from build123d import *

# Parameters (mm, degrees)
SKETCH2_R           = 19.15
BOSS_EXTRUDE1_DEPTH = 25.15
SKETCH3_R           = 1.5
SKETCH3_R_2         = 3.7
CUT_EXTRUDE1_DEPTH  = 5.15
SKETCH4_R           = 7.5
BOSS_EXTRUDE2_DEPTH = 4.5
SKETCH5_R           = 4
CUT_EXTRUDE2_DEPTH  = 4.5
FILLET1_R           = 1


with BuildPart() as part:
    # Sketch2 → Boss-Extrude1 (new body)
    with BuildSketch(Plane.XY):
        with Locations(Location((0, 0, 0), (0, 0, 180))):
            Circle(SKETCH2_R)
    extrude(amount=BOSS_EXTRUDE1_DEPTH)

    # Sketch3 → Cut-Extrude1 (cut)
    with BuildSketch(Plane.XY.offset(25.15)):
        with Locations((11.66726189, 11.66726189)):
            Circle(SKETCH3_R)
        with Locations((-11.66726189, -11.66726189)):
            Circle(SKETCH3_R)
        with Locations((11.66726189, -11.66726189)):
            Circle(SKETCH3_R)
        with Locations((-11.66726189, 11.66726189)):
            Circle(SKETCH3_R)
        with Locations((0, 19.15)):
            Circle(SKETCH3_R_2)
        with Locations((0, -19.15)):
            Circle(SKETCH3_R_2)
        with Locations((-19.15, 0)):
            Circle(SKETCH3_R_2)
        with Locations((19.15, 0)):
            Circle(SKETCH3_R_2)
    extrude(amount=-CUT_EXTRUDE1_DEPTH, mode=Mode.SUBTRACT)

    # Sketch4 → Boss-Extrude2 (add)
    with BuildSketch(Plane.XY.offset(25.15)):
        Circle(SKETCH4_R)
    extrude(amount=BOSS_EXTRUDE2_DEPTH)

    # Sketch5 → Cut-Extrude2 (cut)
    with BuildSketch(Plane.XY.offset(29.65)):
        Circle(SKETCH5_R)
    extrude(amount=-CUT_EXTRUDE2_DEPTH, mode=Mode.SUBTRACT)

    # Fillet1
    fillet1_edges = [part.edges().sort_by_distance(p)[0] for p in [
        (13.54109486, 13.54109486, 25.15),
        (-7.5, 0, 29.65),
        (-13.54109486, 13.54109486, 25.15),
        (-13.54109486, -13.54109486, 25.15),
        (13.54109486, -13.54109486, 25.15),
    ]]
    fillet(fillet1_edges, radius=FILLET1_R)


solid = part.part
Check sheet for the modelled part. Datum: model origin and axes. Units: mm. A direction names the side the tool comes from. Give positions to 0.01 mm unless a question says otherwise; leave off trailing zeros. Loops run counter-clockwise (first coordinate to the right, second up) from the corner with the lowest first, then second, coordinate; pieces in that order, holes last. Notation, with made-up numbers: M 72.25,69 L 119.25,69 A16 ccw 119.25,79 Z; hole C -16,-11 d7. An arc over 180 degrees is marked long. Return JSON: item names as keys, results as strings. Group by question number.
1. Mould release check, pull along Y, two halves, no side actions. Record for faces 1 (the cylindrical face through (-8.837, 16.989, 11.906)), 2 (the flat face through (18, 0, 20)), 3 (the flat face through (0, 18, 20)): released by +Y, released by -Y, zero draft, split by the parting line, or undercut.
2. Thickness scan on L1, parallel to Z at x = 9, y = 6; L2, parallel to Y at x = -2, z = 26; L3, parallel to X at y = 7, z = 6.25. Record the ranges inside material, lowest first.
3. Go/stop test with flat-tipped pins: pin 1 (4 mm diameter, centred on x = -14, y = 15, fed in from +Z); pin 2 (0.9 mm diameter, centred on x = -12, y = -11.5, fed in from +Z); pin 3 (1 mm diameter, centred on x = 13.5, z = 15, fed in from -Y). Record where each tip stops, or that it passes through.
4. Tool access check on faces 4 (the flat face through (-18, 0, 20)), 5 (the flat face through (0, -18, 20)), 6 (the cylindrical face through (15.45, 0.08, 22.61)), 7 (the flat face through (-12, 12, 20)). Record the directions out of +Z, -Z, +X, -X, +Y, -Y that give a thin tool (end or side, any length) a straight path to the whole face; none if there is none.
5. Cross-section at A-A on y = 0. Record the boundary of the cut face in (x, z), plus the area to 3 significant figures.
6. Cross-section at C-C on z = 5.5. Record the boundary of the cut face in (x, y).
Return value:
{
 "1": {"face 1": "split by the parting line", "face 2": "undercut", "face 3": "zero draft"},
 "2": {"L1": "0 to 25.15", "L2": "-7.23 to -3.46, 3.46 to 7.23", "L3": "-17.82 to 17.82"},
 "3": {"pin 1": "z = 25.08", "pin 2": "z = 20", "pin 3": "y = -14.06"},
 "4": {"face 4": "+Z, -X", "face 5": "+Z, -Y", "face 6": "+Z, +X", "face 7": "+Z"},
 "5": {"outline": "M -19.15,0 L 19.15,0 L 19.15,20 L 15.45,20 L 15.45,25.15 L 7.5,25.15 L 7.5,28.65 A1 ccw 6.5,29.65 L 4,29.65 L 4,25.15 L -4,25.15 L -4,29.65 L -6.5,29.65 A1 ccw -7.5,28.65 L -7.5,25.15 L -15.45,25.15 L -15.45,20 L -19.15,20 Z", "area": "956 mm^2"},
 "6": {"outline": "C 0,0 d38.3"}
}
